```python
from build123d import *

# Parameters (mm, degrees)
SKETCH_1_R          = 14.5
EXTRUDE_1_DEPTH     = 18
SKETCH_2_W          = 1
SKETCH_2_H          = 2.5
SKETCH_3_R          = 7.5
CUT_EXTRUDE_1_DEPTH = 5.85
SKETCH_4_R          = 2.5
CUT_EXTRUDE_2_DEPTH = 18
SKETCH_5_R          = 4
CUT_EXTRUDE_3_DEPTH = 18


with BuildPart() as part:
    # 草图1 → 凸台-拉伸1 (new, symmetric)
    with BuildSketch(Plane(origin=(0, 0, 0), x_dir=(1, 0, 0), z_dir=(0, 1, 0))):
        with Locations(Location((0, 0, 0), (0, 0, 270))):
            Circle(SKETCH_1_R)
    extrude(amount=EXTRUDE_1_DEPTH, both=True)

    # 草图2 → 切除-旋转1 (revolve, cut)
    with BuildSketch(Plane(origin=(0, 0, 0), x_dir=(0, 0, -1), z_dir=(1, 0, 0)), mode=Mode.PRIVATE) as cut_revolve_1_sk:
        with Locations((14, -4.35)):
            Rectangle(SKETCH_2_W, SKETCH_2_H)
        with Locations((14, 4.85)):
            Rectangle(SKETCH_2_W, SKETCH_2_H)
    revolve(cut_revolve_1_sk.sketch.rotate(Axis((0, 24.456426369, 0), (0, -1, 0)), 180), axis=Axis((0, 24.456426369, 0), (0, -1, 0)), mode=Mode.SUBTRACT)

    # 草图3 → 切除-拉伸1 (cut, symmetric)
    with BuildSketch(Plane(origin=(0, 0, 0), x_dir=(1, 0, 0), z_dir=(0, 1, 0))):
        with Locations(Location((0, 0, 0), (0, 0, 270))):
            Circle(SKETCH_3_R)
    extrude(amount=CUT_EXTRUDE_1_DEPTH, both=True, mode=Mode.SUBTRACT)

    # 草图4 → 切除-拉伸2 (cut)
    with BuildSketch(Plane(origin=(0, 0, 0), x_dir=(1, 0, 0), z_dir=(0, 1, 0))):
        with Locations(Location((0, 0, 0), (0, 0, 90))):
            Circle(SKETCH_4_R)
    extrude(amount=CUT_EXTRUDE_2_DEPTH, mode=Mode.SUBTRACT)

    # 草图5 → 切除-拉伸3 (cut)
    with BuildSketch(Plane(origin=(0, 0, 0), x_dir=(1, 0, 0), z_dir=(0, 1, 0))):
        with Locations(Location((0, 0, 0), (0, 0, 270))):
            Circle(SKETCH_5_R)
    extrude(amount=-CUT_EXTRUDE_3_DEPTH, mode=Mode.SUBTRACT)


solid = part.part
```
Geometry: final body of the model. Coordinates: model frame, mm. A direction names the side the tool comes from. Round coordinates to 2 decimals unless told otherwise and drop trailing zeros. Order: outer loops, then holes, each group sorted by start corner. A loop starts at its lowest first (then second) coordinate and runs counter-clockwise, first axis right, second up. Notation, with made-up numbers: M -37,-3.75 L -29,-3.75 A18 ccw -29,0.25 Z; hole C -29,17 d3. An arc over 180 degrees is marked long. Use one line per item in the form item = value. Start each with the question number.
Q1. Pin query (flat end, axial travel): pin 1 Ø4 at (x, y) = (10.5, -6) entering from -Z; pin 2 Ø2 at (x, y) = (-2, -3.5) entering from +Z; pin 3 Ø10 at (x, y) = (-10.5, -3) entering from +Z; pin 4 Ø9 at (x, z) = (0, 0) entering from -Y. Return the tip coordinate at first contact, or that it passes through.
Q2. Mould query, pull axis Z, two halves, no side actions, for faces 3 (the face through (-5.554, 12.133, 13.394)), 4 (the face through (-3.905, -11.84, -0.867)), 5 (the face through (10, 6.1, -10)). Classes: +Z half, -Z half, draft (parallel to the pull), parting line (faces both ways), or undercut.
Q3. Cut plane D-D (z = 9). Return loops of the section in (x, y).
Q4. Material intervals for line 1 (Y direction, x = 9.75, z = 9.75); line 2 (X direction, y = 2, z = 0); line 3 (X direction, y = -14.75, z = 0), sorted ascending. Write a range as [from, to].
Q5. Access query for faces 1 (the face through (10, -3.1, -10)), 2 (the face through (-3, -18, 3)). Directions: +Z, -Z, +X, -X, +Y, -Y. A direction counts if a zero-diameter tool reaches every point of the face in a straight line with its end or side. Return the directions, or none.
Q6. Cut plane C-C (y = -15). Return loops of the section in (x, z), and give its area (3 significant figures).
Geometry results:
q1.pin_1 = -11.75
q1.pin_2 = 14.46
q1.pin_3 = 13.42
q1.pin_4 = -18
q2.face_3 = parting line
q2.face_4 = undercut
q2.face_5 = draft
q3.outline = M -11.37,-18 L 11.37,-18 L 11.37,-5.6 L 10.06,-5.6 L 10.06,-3.1 L 11.37,-3.1 L 11.37,3.6 L 10.06,3.6 L 10.06,6.1 L 11.37,6.1 L 11.37,18 L -11.37,18 L -11.37,6.1 L -10.06,6.1 L -10.06,3.6 L -11.37,3.6 L -11.37,-3.1 L -10.06,-3.1 L -10.06,-5.6 L -11.37,-5.6 Z
q4.line_1 = [-18, -5.6], [-3.1, 3.6], [6.1, 18]
q4.line_2 = [-14.5, -7.5], [7.5, 14.5]
q4.line_3 = [-14.5, -4], [4, 14.5]
q5.face_1 = none
q5.face_2 = +Z, -Z, +X, -X, -Y
q6.outline = C 0,0 d29; hole C 0,0 d8
q6.area = 610 mm^2
